from build123d import *

# Parameters (mm, degrees)
F0_W           = 6.35
F0_H           = 142.875
F1_DEPTH       = 38.1
F3_D           = 2.7051
F3_DEPTH       = 15.0876
F3_TIP         = 0.8126940303
F6_D           = 2.2606
F6_DEPTH       = 13.7414
F6_TIP         = 0.6791527577
F6_ON_F4_D     = 2.2606
F6_ON_F4_DEPTH = 13.7414
F6_ON_F4_TIP   = 0.6791527577


with BuildPart() as f1:
    # F0 (on Top) → F1 (new body)
    with BuildSketch(Plane.XY):
        Rectangle(F0_W, F0_H)
    extrude(amount=F1_DEPTH)

    # F3
    with Locations(Plane(origin=(0, 0, 0), x_dir=(1, 0, 0), z_dir=(0, 0, -1))):
        with Locations((0, 46.0375), (0, -46.0375)):
            Hole(F3_D / 2, depth=F3_DEPTH)
            with Locations((0, 0, -(F3_DEPTH + F3_TIP / 2))):  # 118° drill point
                Cone(0, F3_D / 2, F3_TIP, mode=Mode.SUBTRACT)

    # F6
    with Locations(Plane.XZ.offset(71.4375)):
        with Locations((0, 25.4), (0, 12.7)):
            Hole(F6_D / 2, depth=F6_DEPTH)
            with Locations((0, 0, -(F6_DEPTH + F6_TIP / 2))):  # 118° drill point
                Cone(0, F6_D / 2, F6_TIP, mode=Mode.SUBTRACT)

    # F6 on F4
    with Locations(Plane(origin=(0, 71.4375, 0), x_dir=(-1, 0, 0), z_dir=(0, 1, 0))):
        with Locations((0, 31.75), (0, 6.35)):
            Hole(F6_ON_F4_D / 2, depth=F6_ON_F4_DEPTH)
            with Locations((0, 0, -(F6_ON_F4_DEPTH + F6_ON_F4_TIP / 2))):  # 118° drill point
                Cone(0, F6_ON_F4_D / 2, F6_ON_F4_TIP, mode=Mode.SUBTRACT)


solid = f1.part
Design review of the part built by this model. Coordinates are the model's own, in mm. A direction names the side the tool comes from. Coordinates: 2 decimals unless noted, no trailing zeros. Loops run counter-clockwise (first coordinate to the right, second up) from the corner with the lowest first, then second, coordinate; pieces in that order, holes last. Notation, with made-up numbers: (-13.75, 77) - (28.25, 77) arc R29 ccw to (28.25, 97) - close; hole circle Ø8 at (-18, 33.5). An arc over 180 degrees is marked (long way). Use CSV: the item, a comma, the result in double quotes. Start each with the question number.
1. Clearance check with flat-ended pins moving along their axes: pin 1 (1.8 mm diameter, centred on x = 0, z = 12.7, fed in from -Y); pin 2 (1.8 mm diameter, centred on x = 0, z = 31.75, fed in from +Y); pin 3 (2 mm diameter, centred on x = 0, y = 46.04, fed in from -Z). State where each tip first meets the part, or that it passes through.
2. Mouldability with a two-part tool opening along Y and no side actions: class faces 1 (the cylindrical face through (-0.15, 64.47, 32.87)), 2 (the conical face through (-0.186, -45.895, 15.759)), 3 (the conical face through (0.108, 46.246, 15.759)), 4 (the conical face through (0.026, 57.135, 6.545)) as released by +Y, released by -Y, zero draft, split by the parting line, or undercut.
3. To check wall thickness, follow probe 1 along Z at (x, y) = (0, -63.25); probe 2 along Y at (x, z) = (0.75, 12.5); probe 3 along X at (y, z) = (-66.25, 12.7) (3 decimals). State the ranges of each line that lie inside material, in increasing order.
4. Add section A-A on y = 59. Give the boundary of the cut face in (x, z) (3 decimals).
5. For faces 5 (the cylindrical face through (-0.727, -47.178, 7.649)), 6 (the cylindrical face through (0.15, -64.47, 13.82)), 7 (the cylindrical face through (-0.15, 64.47, 7.47)), list the 3-axis set-ups (+Z, -Z, +X, -X, +Y, -Y) from which the entire face can be reached by the end or side of a thin tool; tool diameter is ignored.
Resolved:
1,pin 1,"y = -57.56"
1,pin 2,"y = 57.56"
1,pin 3,"z = 15.3"
2,face 1,"zero draft"
2,face 2,"undercut"
2,face 3,"undercut"
2,face 4,"released by +Y"
3,probe 1,"0 to 11.57, 13.83 to 24.27, 26.53 to 38.1"
3,probe 2,"-57.48 to -47.16, -44.91 to 44.91, 47.16 to 71.44"
3,probe 3,"-3.175 to -1.13, 1.13 to 3.175"
4,outline,"(-3.175, 0) - (3.175, 0) - (3.175, 38.1) - (-3.175, 38.1) - close; hole circle Ø2.261 at (0, 6.35); hole circle Ø2.261 at (0, 31.75)"
5,face 5,"-Z"
5,face 6,"-Y"
5,face 7,"+Y"
